from build123d import *

# Parameters (mm, degrees)
F0_R     = 7.5
F1_DEPTH = 3
F2_R     = 4
F3_DEPTH = 60
F4_R     = 7.5
F5_DEPTH = 3
F6_R     = 2


with BuildPart() as f1:
    # F0 (on Top) → F1 (new body)
    with BuildSketch(Plane.XY):
        Circle(F0_R)
    extrude(amount=F1_DEPTH)

    # F2 (on face) → F3 (join)
    with BuildSketch(Plane.XY.offset(3)):
        Circle(F2_R)
    extrude(amount=F3_DEPTH)

    # F4 (on face) → F5 (join)
    with BuildSketch(Plane.XY.offset(63)):
        Circle(F4_R)
    extrude(amount=F5_DEPTH)

    # F6
    f6_edges = [f1.edges().sort_by_distance(p)[0] for p in [
        (-7.5, 0, 66),
        (-7.5, 0, 0),
    ]]
    fillet(f6_edges, radius=F6_R)


solid = f1.part
Check sheet for the modelled part. Datum: model origin and axes. Units: mm. A direction names the side the tool comes from. Round coordinates to 2 decimals unless told otherwise and drop trailing zeros. Loops run counter-clockwise (first coordinate to the right, second up) from the corner with the lowest first, then second, coordinate; pieces in that order, holes last. Notation, with made-up numbers: M -28,48.5 L -2,48.5 A19 cw -2,65.5 Z; hole C 22,-12 d3. An arc over 180 degrees is marked long. One line per item, written item: value.
(1) Sectioned sample at A-A, the plane x = 0. Record the cut outline in (y, z).
Computed values:
outline: M -7.5,2 A2 ccw -5.5,0 L 5.5,0 A2 ccw 7.5,2 L 7.5,3 L 4,3 L 4,63 L 7.5,63 L 7.5,64 A2 ccw 5.5,66 L -5.5,66 A2 ccw -7.5,64 L -7.5,63 L -4,63 L -4,3 L -7.5,3 Z
(2) Depth check by flat-ended pin: pin 1 Ø6 at (x, z) = (4, 15) entering from -Y; pin 2 Ø3 at (y, z) = (5, 11.5) entering from +X; pin 3 Ø8 at (x, z) = (-1.5, 38) entering from -Y. Enter the tip coordinate at first touch or a pass-through.
Computed values:
pin 1: stops at y = -3.87
pin 2: stops at x = 1.94
pin 3: stops at y = -4
(3) Release check for a two-part mould opening along Z. For faces 3 (the face through (-0.867, -3.905, 32.58)), 4 (the face through (3, -3, 63)), 5 (the face through (-7.493, 0.33, 63.493)), 6 (the face through (0, 0, 0)) record: +Z half, -Z half, draft (parallel to the pull), parting line (faces both ways), or undercut.
Computed values:
face 3: undercut
face 4: undercut
face 5: draft
face 6: -Z half
(4) Sectioned sample at C-C, the plane z = 58. Record the cut outline in (x, y), then the cut area to 3 significant figures.
Computed values:
outline: C 0,0 d8
area: 50.3 mm^2
(5) Access from +Z, -Z, +X, -X, +Y, -Y to the whole of each face (thin tool, end or side, straight path). Record for faces 1 (the face through (3, -3, 3)), 2 (the face through (0, 0, 66)).
Computed values:
face 1: none
face 2: +Z, +X, -X, +Y, -Y
(6) Thickness scan on line 1 (Z direction, x = -5.25, y = 2); line 2 (Z direction, x = -4.5, y = 5); line 3 (Y direction, x = 0.25, z = 19). Record the ranges inside material, lowest first.
Computed values:
line 1: z = 0 to 3, 63 to 66
line 2: z = 0.42 to 3, 63 to 65.58
line 3: y = -3.99 to 3.99
